from build123d import *

# Parameters (mm, degrees)
SKETCH1_R                 = 17.78
SKETCH1_R_2               = 6.35
BOSS_EXTRUDE1_DEPTH       = 3.175
TAP_DRILL_FOR_4_40_TAP1_D = 2.2606


with BuildPart() as part:
    # Sketch1 → Boss-Extrude1 (new body)
    with BuildSketch(Plane(origin=(0, 0, 0), x_dir=(1, 0, 0), z_dir=(0, 1, 0))):
        Circle(SKETCH1_R)
        Circle(SKETCH1_R_2, mode=Mode.SUBTRACT)
    extrude(amount=BOSS_EXTRUDE1_DEPTH)

    # Tap Drill for #4-40 Tap1 (through all)
    with Locations(Plane(origin=(0, 0, 0), x_dir=(-1, 0, 0), z_dir=(0, -1, 0))):
        with Locations((0, -10.16), (-8.798818102, -5.08), (-8.798818102, 5.08), (0, 10.16), (8.798818102, 5.08), (8.798818102, -5.08)):
            Hole(TAP_DRILL_FOR_4_40_TAP1_D / 2)


solid = part.part
Design review of the part built by this model. Coordinates are the model's own, in mm. Coordinates: 2 decimals unless noted, no trailing zeros. Order: outer loops, then holes, each group sorted by start corner. A loop starts at its lowest first (then second) coordinate and runs counter-clockwise, first axis right, second up.
Item 1: The part is to be moulded in two halves that separate along Z. For faces 1 (the cylindrical face through (-9.632, 1.61, -5.844)), 2 (the flat face through (8, 0, 0)), 3 (the cylindrical face through (-0.245, 1.61, -9.057)), 4 (the cylindrical face through (-3.85, 1.57, 17.36)), say which applies: pulls with the +Z half, pulls with the -Z half, needs draft (parallel to the pull), parting line crosses it, or undercut.
Item 2: Take a section at A-A, the plane x = 0. Write out the cut boundary in (y, z) (3 decimals).
Item 3: Take a section at B-B, the plane z = 0. Write out the cut boundary in (x, y) (3 decimals).
Item 4: For pin 1 Ø1.5 at (y, z) = (1.5, 5.5) entering from +X; pin 2 Ø1.5 at (x, y) = (3, 2) entering from -Z; pin 3 Ø1.5 at (y, z) = (2.5, 10) entering from -X, all flat-tipped, find the tip position at first contact; note any pin that passes through.
Item 5: For line 1 (Z direction, x = 0, y = 0.85); line 2 (X direction, y = 1.65, z = -5); line 3 (X direction, y = 1.5, z = -5.08), list the stretches that pass through material, from the lowest coordinate up.
Item 6: Take a section at C-C, the plane y = 1.6. Write out the cut boundary in (x, z), then the cut area to 3 significant figures.
Item 7: Take a section at D-D, the plane z = -5.08. Write out the cut boundary in (x, y) (3 decimals), then the cut area to 3 significant figures.
The answers:
1. face 1: undercut
1. face 2: needs draft
1. face 3: undercut
1. face 4: parting line crosses it
2. outline: (0, -17.78) - (3.175, -17.78) - (3.175, -11.29) - (0, -11.29) - close; (0, -9.03) - (3.175, -9.03) - (3.175, -6.35) - (0, -6.35) - close; (0, 6.35) - (3.175, 6.35) - (3.175, 9.03) - (0, 9.03) - close; (0, 11.29) - (3.175, 11.29) - (3.175, 17.78) - (0, 17.78) - close
3. outline: (-17.78, 0) - (-6.35, 0) - (-6.35, 3.175) - (-17.78, 3.175) - close; (6.35, 0) - (17.78, 0) - (17.78, 3.175) - (6.35, 3.175) - close
4. pin 1: stops at x = 17.13
4. pin 2: stops at z = -17.64
4. pin 3: stops at x = -15.18
5. line 1: z = -17.78 to -11.29, -9.03 to -6.35, 6.35 to 9.03, 11.29 to 17.78
5. line 2: x = -17.06 to -9.93, -7.67 to -3.91, 3.91 to 7.67, 9.93 to 17.06
5. line 3: x = -17.04 to -9.93, -7.67 to -3.81, 3.81 to 7.67, 9.93 to 17.04
6. outline: circle Ø35.56 at (0, 0); hole circle Ø2.26 at (-8.8, -5.08); hole circle Ø2.26 at (-8.8, 5.08); hole circle Ø12.7 at (0, 0); hole circle Ø2.26 at (0, -10.16); hole circle Ø2.26 at (0, 10.16); hole circle Ø2.26 at (8.8, -5.08); hole circle Ø2.26 at (8.8, 5.08)
6. area: 842 mm2
7. outline: (-17.039, 0) - (-9.929, 0) - (-9.929, 3.175) - (-17.039, 3.175) - close; (-7.669, 0) - (-3.81, 0) - (-3.81, 3.175) - (-7.669, 3.175) - close; (3.81, 0) - (7.669, 0) - (7.669, 3.175) - (3.81, 3.175) - close; (9.929, 0) - (17.039, 0) - (17.039, 3.175) - (9.929, 3.175) - close
7. area: 69.6 mm2
